Input: part model. Units: mm. Frame: model coordinates. A direction names the side the tool comes from. Coordinates: 2 decimals unless noted, no trailing zeros. Write each loop counter-clockwise with the first axis right and the second up, starting at its lowest first coordinate (ties: lowest second). Pieces come first, ordered by that corner, then holes.
from build123d import *

# Parameters (mm, degrees)
SKETCH_1_W               = 43
SKETCH_1_H               = 20
EXTRUDE_1_DEPTH          = 3
CUT_EXTRUDE_1_DEPTH      = 24.900836805
CUT_EXTRUDE_1_DEPTH_BACK = 24.900836805
SKETCH_2_R               = 1
SKETCH_3_R               = 7.9
EXTRUDE_2_DEPTH          = 12
FILLET_1_R               = 0.5
SKETCH_5_R               = 6.9
CUT_EXTRUDE_2_DEPTH      = 0.3
EXTRUDE_3_DEPTH          = 3.5
FILLET_2_R               = 0.5


with BuildPart() as part:
    # 스케치1 → 보스-돌출1 (new body)
    with BuildSketch(Plane.XY):
        Rectangle(SKETCH_1_W, SKETCH_1_H)
    extrude(amount=EXTRUDE_1_DEPTH)

    # 스케치2 → 컷-돌출1 (cut, two sides: drawn at the far end of the back side and taken through both)
    with BuildSketch(Plane.XY.offset(3).offset(-CUT_EXTRUDE_1_DEPTH_BACK)):
        with Locations((20, 8.5)):
            Circle(SKETCH_2_R)
        with Locations(Location((-20, 8.5, 0), (0, 0, 180))):
            Circle(SKETCH_2_R)
        with Locations(Location((20, -8.5, 0), (0, 0, 180))):
            Circle(SKETCH_2_R)
        with Locations((-20, -8.5)):
            Circle(SKETCH_2_R)
    extrude(amount=CUT_EXTRUDE_1_DEPTH + CUT_EXTRUDE_1_DEPTH_BACK, mode=Mode.SUBTRACT)

    # 스케치3 → 보스-돌출2 (add)
    with BuildSketch(Plane.XY.offset(3)):
        with Locations(Location((11.4, 0, 0), (0, 0, 180))):
            Circle(SKETCH_3_R)
        with Locations(Location((-11.4, 0, 0), (0, 0, 180))):
            Circle(SKETCH_3_R)
    extrude(amount=EXTRUDE_2_DEPTH)

    # 필렛1
    fillet_1_edges = [part.edges().sort_by_distance(p)[0] for p in [
        (19.3, 0, 15),
        (-3.5, 0, 15),
    ]]
    fillet(fillet_1_edges, radius=FILLET_1_R)

    # 스케치5 → 컷-돌출2 (cut)
    with BuildSketch(Plane.XY.offset(15)):
        with Locations((-11.4, 0)):
            Circle(SKETCH_5_R)
        with Locations((11.4, 0)):
            Circle(SKETCH_5_R)
    extrude(amount=-CUT_EXTRUDE_2_DEPTH, mode=Mode.SUBTRACT)

    # 스케치6 → 보스-돌출3 (add)
    with BuildSketch(Plane.XY.offset(3)):
        with BuildLine():
            Line((-3.2, 9.325), (3.2, 9.325))
            ThreePointArc((3.2, 9.325), (5.525, 7), (3.2, 4.675))
            Line((3.2, 4.675), (-3.2, 4.675))
            ThreePointArc((-3.2, 4.675), (-5.525, 7), (-3.2, 9.325))
        make_face()
    extrude(amount=EXTRUDE_3_DEPTH)

    # 필렛2
    fillet_2_edges = [part.edges().sort_by_distance(p)[0] for p in [
        (-5.525, 7, 6.5),
        (0, 4.675, 6.5),
        (5.525, 7, 6.5),
        (0, 9.325, 6.5),
    ]]
    fillet(fillet_2_edges, radius=FILLET_2_R)


solid = part.part
Item 1: Pull-direction query (Y, two-part tool) for faces 1 (the face through (0, 4.675, 4)), 2 (the face through (-5.524, 6.949, 4.479)), 3 (the face through (0, 0, 0)), 4 (the face through (-20.13, -7.51, 1.48)); classes: released by +Y, released by -Y, zero draft, split by the parting line, or undercut.
Item 2: Section query D-D, the plane z = 13. Return loops of the section in (x, y), then the cut area to 3 significant figures.
Item 3: Pin query (flat end, axial travel): pin 1 Ø1.8 at (x, y) = (-20, -8.5) entering from -Z; pin 2 Ø3 at (x, z) = (5.5, 9.5) entering from +Y; pin 3 Ø2 at (y, z) = (-5.5, 5) entering from -X; pin 4 Ø3 at (x, y) = (2, -4.5) entering from +Z. Return the tip coordinate at first contact, or that it passes through.
Item 4: Section query B-B, the plane x = 20. Return loops of the section in (y, z), then the cut area to 3 significant figures.
Item 5: Section query C-C, the plane x = -11.4. Return loops of the section in (y, z), then the cut area to 3 significant figures.
Item 6: Section query A-A, the plane z = 5.25. Return loops of the section in (x, y) (3 decimals).
Item 7: Access query for faces 5 (the face through (-19.87, 7.51, 1.48)), 6 (the face through (-11, 0, 14.7)), 7 (the face through (0, 7, 6.5)). Directions: +Z, -Z, +X, -X, +Y, -Y. A direction counts if a zero-diameter tool reaches every point of the face in a straight line with its end or side. Return the directions, or none.
Item 8: Material intervals for line 1 (Y direction, x = -20, z = 1.9); line 2 (X direction, y = -0.25, z = 10.5); line 3 (Z direction, x = 2.5, y = -7), sorted ascending.
The answers:
1. face 1: released by -Y
1. face 2: undercut
1. face 3: zero draft
1. face 4: undercut
2. outline: circle Ø15.8 at (-11.4, 0); circle Ø15.8 at (11.4, 0)
2. area: 392 mm2
3. pin 1: passes through
3. pin 2: stops at y = 6.56
3. pin 3: stops at x = -17.89
3. pin 4: stops at z = 3
4. outline: (-10, 0) - (-9.5, 0) - (-9.5, 3) - (-10, 3) - close; (-7.5, 0) - (7.5, 0) - (7.5, 3) - (-7.5, 3) - close; (9.5, 0) - (10, 0) - (10, 3) - (9.5, 3) - close
4. area: 48.0 mm2
5. outline: (-10, 0) - (10, 0) - (10, 3) - (7.9, 3) - (7.9, 14.5) arc R0.5 ccw to (7.4, 15) - (6.9, 15) - (6.9, 14.7) - (-6.9, 14.7) - (-6.9, 15) - (-7.4, 15) arc R0.5 ccw to (-7.9, 14.5) - (-7.9, 3) - (-10, 3) - close
5. area: 245 mm2
6. outline: circle Ø15.8 at (-11.4, 0); (-3.2, 4.675) - (3.2, 4.675) arc R2.325 ccw to (3.2, 9.325) - (-3.2, 9.325) arc R2.325 ccw to start; circle Ø15.8 at (11.4, 0)
7. face 5: +Z, -Z
7. face 6: +Z
7. face 7: +Z, +Y
8. line 1: y = -10 to -9.5, -7.5 to 7.5, 9.5 to 10
8. line 2: x = -19.3 to -3.5, 3.5 to 19.3
8. line 3: z = 0 to 3
